```python
from build123d import *

# Parameters (mm, degrees)
SKETCH1_W           = 144.78
SKETCH1_H           = 206.248
EXTRUDE1_DEPTH      = 252.4252
SKETCH7_W           = 125.73
SKETCH7_H           = 196.723
EXTRUDE5_DEPTH      = 35.64418
EXTRUDE2_DEPTH      = 42.08
EXTRUDE2_DEPTH_BACK = 273.8502
SKETCH4_W           = 113.03
SKETCH4_H           = 142.748
SKETCH10_W          = 113.03
SKETCH10_H          = 2.921
SKETCH10_H_2        = 45.974
EXTRUDE8_DEPTH      = 264.16
SKETCH11_W          = 113.03
SKETCH11_H          = 2.921
EXTRUDE9_DEPTH      = 21.59
FILLET1_R           = 2.54
SKETCH2_R           = 245.618
EXTRUDE4_DEPTH      = 230
SKETCH12_W          = 125.73
SKETCH12_H          = 43.053
EXTRUDE10_DEPTH     = 21.36938
SKETCH14_W          = 132.74265683
SKETCH14_H          = 39.732066683
CUT_EXTRUDE1_DEPTH  = 15.623999994
SKETCH15_W          = 144.34776975
SKETCH15_H          = 23.27915683
CUT_EXTRUDE2_DEPTH  = 15.623999994


with BuildPart() as part:
    # Sketch1 → Extrude1 (new body)
    with BuildSketch(Plane.XY):
        with Locations((25.4, -16.764)):
            Rectangle(SKETCH1_W, SKETCH1_H)
    extrude(amount=EXTRUDE1_DEPTH)

    # Sketch7 → Extrude5 (add)
    with BuildSketch(Plane.XY.offset(252.4252)):
        with Locations((25.4, -21.5265)):
            Rectangle(SKETCH7_W, SKETCH7_H)
    extrude(amount=EXTRUDE5_DEPTH)

    # Sketch4 → Extrude2 (cut, two sides: drawn at the far end of the back side and taken through both)
    with BuildSketch(Plane.XY.offset(252.4252).offset(-EXTRUDE2_DEPTH_BACK)):
        with Locations((25.4, 0)):
            Rectangle(SKETCH4_W, SKETCH4_H)
    extrude(amount=EXTRUDE2_DEPTH + EXTRUDE2_DEPTH_BACK, mode=Mode.SUBTRACT)

    # Sketch10 → Extrude8 (cut)
    with BuildSketch(Plane(origin=(0, 0, 0), x_dir=(-1, 0, 0), z_dir=(0, 0, -1))):
        with Locations((-25.4, 72.8345)):
            Rectangle(SKETCH10_W, SKETCH10_H)
        with Locations((-25.4, -94.361)):
            Rectangle(SKETCH10_W, SKETCH10_H_2)
    extrude(amount=-EXTRUDE8_DEPTH, mode=Mode.SUBTRACT)

    # Sketch11 → Extrude9 (cut)
    with BuildSketch(Plane(origin=(0, 0, 264.16), x_dir=(-1, 0, 0), z_dir=(0, 0, -1))):
        with Locations((-25.4, 72.8345)):
            Rectangle(SKETCH11_W, SKETCH11_H)
    extrude(amount=-EXTRUDE9_DEPTH, mode=Mode.SUBTRACT)

    # Fillet1
    fillet1_edges = [part.edges().sort_by_distance(p)[0] for p in [
        (-31.115, 71.374, 286.90969),
        (-31.115, -71.374, 276.11469),
        (81.915, -71.374, 276.11469),
        (81.915, 71.374, 286.90969),
        (81.915, 74.295, 142.875),
        (-31.115, 74.295, 142.875),
        (81.915, -117.348, 132.08),
        (-31.115, -117.348, 132.08),
    ]]
    fillet(fillet1_edges, radius=FILLET1_R)

    # Sketch2 → Extrude4 (cut)
    with BuildSketch(Plane(origin=(0, 86.36, 0), x_dir=(-1, 0, 0), z_dir=(0, 1, 0))):
        with Locations((-25.4, 0)):
            Circle(SKETCH2_R)
    extrude(amount=-EXTRUDE4_DEPTH, mode=Mode.SUBTRACT)

    # Sketch12 → Extrude10 (cut)
    with BuildSketch(Plane.XY.offset(288.06938)):
        with Locations((25.4, -98.3615)):
            Rectangle(SKETCH12_W, SKETCH12_H)
    extrude(amount=-EXTRUDE10_DEPTH, mode=Mode.SUBTRACT)

    # Sketch14 → Cut-Extrude1 (cut)
    with BuildSketch(Plane(origin=(0, 76.835, 0), x_dir=(1, 0, 0), z_dir=(0, 1, 0))):
        with Locations((21.893671585, -272.291233342)):
            Rectangle(SKETCH14_W, SKETCH14_H)
    extrude(amount=-CUT_EXTRUDE1_DEPTH, mode=Mode.SUBTRACT)

    # Sketch15 → Cut-Extrude2 (cut)
    with BuildSketch(Plane.XZ.offset(76.835)):
        with Locations((25.85194999, 278.339578415)):
            Rectangle(SKETCH15_W, SKETCH15_H)
    extrude(amount=-CUT_EXTRUDE2_DEPTH, mode=Mode.SUBTRACT)


solid = part.part
```
Build history of the part. All positions in model axes, mm. A direction names the side the tool comes from. Round coordinates to 2 decimals unless told otherwise and drop trailing zeros. Write each loop counter-clockwise with the first axis right and the second up, starting at its lowest first coordinate (ties: lowest second). Pieces come first, ordered by that corner, then holes. Notation, with made-up numbers: (42.5, 70) -> (97.5, 70) arc R20 ccw to (97.5, 100) -> close; hole circle Ø2 at (-7.75, 11.25). An arc over 180 degrees is marked (long way). Put each result on its own line as item: value.
Item 1: Flat gauge pins, fed straight in: P1, Ø7, axis at x = 83.5, z = 276, coming from the -Y side; P2, Ø3, axis at x = 25, z = 265.5, coming from the +Y side; P3, Ø5, axis at x = 86.5, z = 263.5, coming from the +Y side. Where does each tip first touch, or does it go through?
Here are the results:
P1: stops at y = -61.21
P2: stops at y = -71.37
P3: stops at y = 61.21
Item 2: Two-plate mould, pull along X, no slides. Class faces 1 (the face through (-37.465, -10, 270)), 2 (the face through (26, -98, 264.16)), 3 (the face through (81.915, -2, 263)), 4 (the face through (24, -119.888, 254)): pulls with the +X half, pulls with the -X half, needs draft (parallel to the pull), parting line crosses it, or undercut.
Here are the results:
face 1: pulls with the -X half
face 2: undercut
face 3: undercut
face 4: needs draft
Item 3: Slice it at B-B, the plane z = 249. Give the cut face in (x, y) (3 decimals), plus the area to 3 significant figures.
Here are the results:
outline: (-46.99, -119.888) -> (97.79, -119.888) -> (97.79, 86.36) -> (-46.99, 86.36) -> close; hole (-31.115, -114.808) arc R2.54 ccw to (-28.575, -117.348) -> (79.375, -117.348) arc R2.54 ccw to (81.915, -114.808) -> (81.915, 71.755) arc R2.54 ccw to (79.375, 74.295) -> (-28.575, 74.295) arc R2.54 ccw to (-31.115, 71.755) -> close
area: 8,200 mm^2
Item 4: Slice it at D-D, the plane x = -8. Give the cut face in (y, z) (3 decimals), plus the area to 3 significant figures.
Here are the results:
outline: (-119.888, 243.336) -> (-117.348, 243.336) -> (-117.348, 264.16) -> (-71.374, 264.16) -> (-71.374, 266.7) -> (-119.888, 266.7) -> close; (74.295, 243.336) -> (86.36, 243.336) -> (86.36, 252.425) -> (74.295, 252.425) -> close
area: 286 mm^2
Item 5: Tool access for faces 5 (the face through (88.265, -10, 270)), 6 (the face through (25, -91, 266.7)), 7 (the face through (26, 74.295, 247)), 8 (the face through (-34, 61.211, 270)), 9 (the face through (26, -117.348, 254)): list every direction of +Z, -Z, +X, -X, +Y, -Y with a clear straight run to the whole face (end or side of a thin tool).
Here are the results:
face 5: +Z, +X, +Y, -Y
face 6: +Z, +X, -X, -Y
face 7: +Z, -Z
face 8: +Z, +X, -X, +Y
face 9: -Z
Item 6: Slice it at C-C, the plane z = 271.5. Give the cut face in (x, y) (3 decimals).
Here are the results:
outline: (-37.465, -61.211) -> (-31.115, -61.211) -> (-31.115, 61.211) -> (-37.465, 61.211) -> close; (81.915, -61.211) -> (88.265, -61.211) -> (88.265, 61.211) -> (81.915, 61.211) -> close
Item 7: Slice it at A-A, the plane y = 58. Give the cut face in (x, z) (3 decimals).
Here are the results:
outline: (-46.99, 234.708) arc R245.618 cw to (-31.115, 239.028) -> (-31.115, 288.069) -> (-37.465, 288.069) -> (-37.465, 252.425) -> (-46.99, 252.425) -> close; (81.915, 239.028) arc R245.618 cw to (97.79, 234.708) -> (97.79, 252.425) -> (88.265, 252.425) -> (88.265, 288.069) -> (81.915, 288.069) -> close
Item 8: Wall check: probe 1 along Y at (x, z) = (25, 252) (3 decimals); probe 2 along X at (y, z) = (-29.5, 254) (3 decimals); probe 3 along X at (y, z) = (-34, 245.5) (3 decimals). Give the ranges that are in metal, low to high. Write a range as from..to.
Here are the results:
probe 1: y = -119.888..-117.348, 74.295..86.36
probe 2: x = -37.465..-31.115, 81.915..88.265
probe 3: x = -46.99..-31.115, 81.915..97.79
